```python
from build123d import *

# Parameters (mm, degrees)
BOSS_EXTRUDE1_DEPTH      = 8.0645
BOSS_EXTRUDE1_DEPTH_BACK = 8.0645
CUT_EXTRUDE1_REACH       = 58.397
SKETCH2_R                = 2.921
CUT_EXTRUDE2_REACH       = 56.482
SKETCH5_R                = 2.921
FILLET1_R                = 2.54


with BuildPart() as part:
    # Sketch1 → Boss-Extrude1 (new, two sides: drawn at the far end of the back side and taken through both)
    with BuildSketch(Plane.XY.offset(-BOSS_EXTRUDE1_DEPTH_BACK)):
        Polygon((0, 0), (2.6924, 0), (2.6924, 38.1), (38.1, 38.1), (38.1, 40.7924), (0, 40.7924), (0, 38.1), align=None)
    extrude(amount=BOSS_EXTRUDE1_DEPTH + BOSS_EXTRUDE1_DEPTH_BACK)

    # Sketch2 → Cut-Extrude1 (cut, up to next)
    with BuildSketch(Plane.ZY, mode=Mode.PRIVATE) as cut_extrude1_sk1:
        with Locations((1.7145, 7.62)):
            Circle(SKETCH2_R)
    cut_extrude1_tool1 = extrude(cut_extrude1_sk1.sketch, amount=-CUT_EXTRUDE1_REACH, mode=Mode.PRIVATE) & part.part
    # Sketch2 → Cut-Extrude1 (cut, up to next)
    with BuildSketch(Plane.ZY, mode=Mode.PRIVATE) as cut_extrude1_sk2:
        with Locations((-1.7145, 23.241)):
            Circle(SKETCH2_R)
    cut_extrude1_tool2 = extrude(cut_extrude1_sk2.sketch, amount=-CUT_EXTRUDE1_REACH, mode=Mode.PRIVATE) & part.part
    add(cut_extrude1_tool1.solids().sort_by_distance((0, 7.62, 1.7145))[0], mode=Mode.SUBTRACT)
    add(cut_extrude1_tool2.solids().sort_by_distance((0, 23.241, -1.7145))[0], mode=Mode.SUBTRACT)

    # Sketch5 → Cut-Extrude2 (cut, up to next)
    with BuildSketch(Plane.XZ.offset(-38.1), mode=Mode.PRIVATE) as cut_extrude2_sk1:
        with Locations(Location((30.48, -1.7145, 0), (0, 0, 270))):
            Circle(SKETCH5_R)
    cut_extrude2_tool1 = extrude(cut_extrude2_sk1.sketch, amount=-CUT_EXTRUDE2_REACH, mode=Mode.PRIVATE) & part.part
    # Sketch5 → Cut-Extrude2 (cut, up to next)
    with BuildSketch(Plane.XZ.offset(-38.1), mode=Mode.PRIVATE) as cut_extrude2_sk2:
        with Locations(Location((15.24, 1.7145, 0), (0, 0, 270))):
            Circle(SKETCH5_R)
    cut_extrude2_tool2 = extrude(cut_extrude2_sk2.sketch, amount=-CUT_EXTRUDE2_REACH, mode=Mode.PRIVATE) & part.part
    add(cut_extrude2_tool1.solids().sort_by_distance((30.48, 38.1, -1.7145))[0], mode=Mode.SUBTRACT)
    add(cut_extrude2_tool2.solids().sort_by_distance((15.24, 38.1, 1.7145))[0], mode=Mode.SUBTRACT)

    # Fillet1
    fillet1_edges = [part.edges().sort_by_distance(p)[0] for p in [
        (0, 40.7924, 0),
        (2.6924, 38.1, 0),
    ]]
    fillet(fillet1_edges, radius=FILLET1_R)


solid = part.part
```
Model file for the job. Use its own axes, mm. A direction names the side the tool comes from. Round coordinates to 2 decimals unless told otherwise and drop trailing zeros. Order: outer loops, then holes, each group sorted by start corner. A loop starts at its lowest first (then second) coordinate and runs counter-clockwise, first axis right, second up. Notation, with made-up numbers: (-36.5, 27) -> (22.5, 27) arc R31 ccw to (22.5, 60) -> close; hole circle Ø11 at (41, 75.5). An arc over 180 degrees is marked (long way). Use one line per item in the form item = value.
Item 1: Cut at A-A, the plane y = 7.62. Write the cut outline in (x, z), and give its area (3 significant figures).
Returned:
outline = (0, -8.06) -> (2.69, -8.06) -> (2.69, -1.21) -> (0, -1.21) -> close; (0, 4.64) -> (2.69, 4.64) -> (2.69, 8.06) -> (0, 8.06) -> close
area = 27.7 mm^2
Item 2: Pull direction Z, two halves, no side cores. Call faces 1 (the face through (0.724, 40.029, 0.113)), 2 (the face through (2, 30, 8.065)), 3 (the face through (1.33, 4.77, 1.08)), 4 (the face through (32.943, 39.427, -3.285)): released by +Z, released by -Z, zero draft, split by the parting line, or undercut.
Returned:
face_1 = zero draft
face_2 = released by +Z
face_3 = undercut
face_4 = undercut
Item 3: Cut at B-B, the plane x = 30.48. Write the cut outline in (y, z), and give its area (3 significant figures).
Returned:
outline = (38.1, -8.06) -> (40.79, -8.06) -> (40.79, -4.64) -> (38.1, -4.64) -> close; (38.1, 1.21) -> (40.79, 1.21) -> (40.79, 8.06) -> (38.1, 8.06) -> close
area = 27.7 mm^2
Item 4: Tool access for faces 5 (the face through (21, 38.1, 0)), 6 (the face through (2, 30, -8.065)): list every direction of +Z, -Z, +X, -X, +Y, -Y with a clear straight run to the whole face (end or side of a thin tool).
Returned:
face_5 = +Z, -Z, +X, -Y
face_6 = -Z, +X, -X, +Y, -Y
Item 5: Cut at D-D, the plane y = 15. Write the cut outline in (x, z).
Returned:
outline = (0, -8.06) -> (2.69, -8.06) -> (2.69, 8.06) -> (0, 8.06) -> close
Item 6: Cut at C-C, the plane z = 3.75. Write the cut outline in (x, y), and give its area (3 significant figures).
Returned:
outline = (0, 0) -> (2.69, 0) -> (2.69, 5.53) -> (0, 5.53) -> close; (0, 9.71) -> (2.69, 9.71) -> (2.69, 35.56) arc R2.54 cw to (5.23, 38.1) -> (13.15, 38.1) -> (13.15, 40.79) -> (2.54, 40.79) arc R2.54 ccw to (0, 38.25) -> close; (17.33, 38.1) -> (38.1, 38.1) -> (38.1, 40.79) -> (17.33, 40.79) -> close
area = 183 mm^2
Item 7: Drill centre lines: line 1 (X direction, y = 20.5, z = -5); line 2 (Y direction, x = 33.5, z = -4.25); line 3 (Y direction, x = 2.5, z = 0). Where is each one in solid material? Low to high.
Returned:
line_1 = 0 to 2.69
line_2 = 38.1 to 40.79
line_3 = 0 to 5.26, 9.98 to 20.88, 25.61 to 40.79
Item 8: Flat gauge pins, fed straight in: pin 1 Ø4 at (x, y) = (6, 25) entering from +Z; pin 2 Ø7.5 at (y, z) = (23.24, -1.71) entering from +X; pin 3 Ø5 at (x, z) = (17, 4) entering from -Y. Where does each tip first touch, or does it go through?
Returned:
pin_1 = through
pin_2 = 2.69
pin_3 = 38.1
